Autodesk Inventor part; units mm, degrees
ref_plane "Work Plane1" through (0, 24.13, 0) normal (0, 1, 0) x (1, 0, 0)
ref_plane "YZ Plane" through (0, 0, 0) normal (1, 0, 0) x (0, 1, 0)
ref_plane "XZ Plane" through (0, 0, 0) normal (0, 1, 0) x (-1, 0, 0)
sketch "Sketch1" plane through (0, 0, 0) normal (0, 1, 0) x (-1, 0, 0)
  circle A0 centre (0, 0) radius 127
  dimension "d0" = 254
extrude "Extrusion1" add sketch "Sketch1" along normal mid plane 7.62
sketch "Sketch2" plane through (0, 3.81, 0) normal (0, 1, 0) x (1, 0, 0)
  line L0 (0, 0) -> (0, -63.5)
  line L1 (12.7, -69.85) -> (-12.7, -69.85)
  line L2 (-12.7, -69.85) -> (-12.7, -57.15)
  line L3 (-12.7, -57.15) -> (12.7, -57.15)
  line L4 (12.7, -57.15) -> (12.7, -69.85)
  line L5 (12.7, -69.85) -> (-12.7, -57.15) construction
  line L6 (-12.7, -69.85) -> (12.7, -57.15) construction
  dimension "d4" = 63.5
  dimension "d5" = 12.7
  dimension "d6" = 25.4
ref_plane "Work Plane1" through (0, 24.13, 0) normal (0, 1, 0) x (1, 0, 0)
sketch "Sketch3" plane through (0, 24.13, 0) normal (0, 1, 0) x (1, 0, 0)
  line L0 (0, 0) -> (0, -50.8)
  line L1 (12.7, -57.15) -> (-12.7, -57.15)
  line L2 (-12.7, -57.15) -> (-12.7, -44.45)
  line L3 (-12.7, -44.45) -> (12.7, -44.45)
  line L4 (12.7, -44.45) -> (12.7, -57.15)
  line L5 (12.7, -57.15) -> (-12.7, -44.45) construction
  line L6 (-12.7, -57.15) -> (12.7, -44.45) construction
  dimension "d8" = 50.8
  dimension "d9" = 12.7
  dimension "d10" = 25.4
loft "Loft1" add profiles "Sketch2", "Sketch3"
sketch "Sketch4" plane through (0, 0, 0) normal (0, 0, 1) x (1, 0, 0)
  line L0 (0, 0) -> (0, 24.13)
  line L1 (12.7, 24.13) -> (-12.7, 24.13)
  line L2 (0, 24.13) -> (0, 21.59)
  line L3 (-12.7, 19.05) -> (12.7, 19.05)
  line L4 (12.7, 19.05) -> (12.7, 24.13)
  line L5 (12.7, 24.13) -> (-12.7, 24.13)
  line L6 (-12.7, 24.13) -> (-12.7, 19.05)
  line L7 (-12.7, 19.05) -> (12.7, 24.13) construction
  line L8 (12.7, 19.05) -> (-12.7, 24.13) construction
  dimension "d15" = 2.54
  dimension "d16" = 25.4
extrude "Extrusion2" add sketch "Sketch4" along normal up to next
mirror "Mirror1" about plane through (0, 0, 0) normal (0, 0, 1) of "Loft1", "Extrusion2"
sketch "Sketch5" plane through (0, 3.81, 0) normal (0, 1, 0) x (1, 0, 0)
  line L0 (0, 0) -> (-122.1674, 0)
  dimension "d19" = 122.1674
hole "Hole1" at (-122.1674, 3.81, 0) direction (0, -1, 0) diameter 4.9784 depth 19.05 tip angle 118
pattern_circular "Circular Pattern1" count 4 over 360 about axis through (0, -10, 0) along (0, 1, 0) of "Hole1"
properties part number "Avi Bay Lid" material "Steel, Alloy"
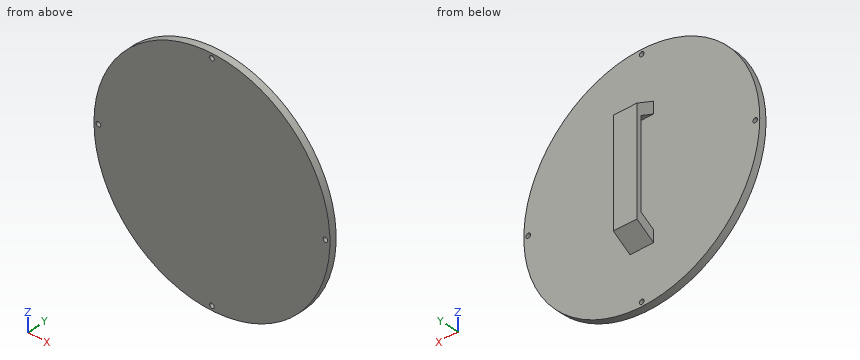
Input: part model. Units: mm. Frame: model coordinates. Coordinates: 2 decimals unless noted, no trailing zeros. Loops run counter-clockwise (first coordinate to the right, second up) from the corner with the lowest first, then second, coordinate; pieces in that order, holes last. Notation, with made-up numbers: M 12.5,70.25 L 68.5,70.25 A10 cw 68.5,78.25 Z; hole C 13.25,39 d6. An arc over 180 degrees is marked long. Use a Markdown table: item, result. Add a question column.
1) Pin query (flat end, axial travel): P1, Ø6.5, axis at x = 122.17, z = 0, coming from the +Y side; P2, Ø3, axis at x = 17, y = 4.5, coming from the -Z side; P3, Ø5.5, axis at x = -122.17, z = 0, coming from the -Y side; P4, Ø2, axis at y = 0.5, z = -92, coming from the +X side. Return the tip coordinate at first contact, or that it passes through.
2) Section B-B, the plane y = 11.5. Return the cut outline in (x, z).
3) Section C-C, the plane x = 22. Return the cut outline in (y, z).
4) Section A-A, the plane z = 54. Return the cut outline in (x, y), plus the area to 3 significant figures.
5) Line query: L1, parallel to Z at x = 0, y = 1; L2, parallel to Y at x = -9.5, z = -16.5; L3, parallel to Y at x = -31, z = -49.5. Output: solid intervals per line, ascending. Write a range as from..to.
Answer below:
| question | item | result |
|---|---|---|
| 1 | P1 | y = 3.81 |
| 1 | P2 | z = -126.03 |
| 1 | P3 | y = -3.81 |
| 1 | P4 | x = 88.59 |
| 2 | outline | M -12.7,-65.04 L 12.7,-65.04 L 12.7,-52.34 L -12.7,-52.34 Z; M -12.7,52.34 L 12.7,52.34 L 12.7,65.04 L -12.7,65.04 Z |
| 3 | outline | M -3.81,-125.08 L 3.81,-125.08 L 3.81,125.08 L -3.81,125.08 Z |
| 4 | outline | M -114.95,-3.81 L 114.95,-3.81 L 114.95,3.81 L -114.95,3.81 Z; M -12.7,8.85 L 12.7,8.85 L 12.7,24.13 L -12.7,24.13 Z |
| 4 | area | 2,140 mm2 |
| 5 | L1 | -127..-124.66, -119.68..119.68, 124.66..127 |
| 5 | L2 | -3.81..3.81, 19.05..24.13 |
| 5 | L3 | -3.81..3.81 |
